Build history of the part. All positions in model axes, mm. Face numbers are marked on the shaded views. A direction names the side the tool comes from. Round coordinates to 2 decimals unless told otherwise and drop trailing zeros. Write each loop counter-clockwise with the first axis right and the second up, starting at its lowest first coordinate (ties: lowest second). Pieces come first, ordered by that corner, then holes.
Item 1: Mould opens along Y. For the marked faces 1, 2 and 3 say: +Y half, -Y half, draft (parallel to the pull), parting line (faces both ways), or undercut.
Item 2: 3-axis set-ups, long thin cutter, end or side, ignore diameter. For the marked faces 4 and 5: which of +Z, -Z, +X, -X, +Y, -Y reach the whole face in a straight line?
Item 3: Band-saw the part on D-D, the plane z = 24.5. Write the cut outline in (x, y) (3 decimals), then the cut area to 3 significant figures.
Item 4: Band-saw the part on A-A, the plane y = -8.5. Write the cut outline in (x, z) (3 decimals).
Item 5: Band-saw the part on B-B, the plane y = 0. Write the cut outline in (x, z) (3 decimals).
Item 6: Band-saw the part on C-C, the plane x = 10. Write the cut outline in (y, z) (3 decimals), then the cut area to 3 significant figures.
Item 7: Drop a flat-ended pin along its axis: pin 1 Ø2 at (x, y) = (-8.5, -17.5) entering from +Z. Give the stop position or say it passes through.
Item 8: Wall check: probe 1 along X at (y, z) = (2, 71.5) (3 decimals); probe 2 along Z at (x, y) = (19.7, 0) (3 decimals). Give the ranges that are in metal, low to high.
```python
from build123d import *

# Parameters (mm, degrees)
SKETCH2_W           = 44.45
SKETCH2_H           = 44.45
SKETCH2_W_2         = 38.1
SKETCH2_H_2         = 38.1
BOSS_EXTRUDE1_DEPTH = 101.6
SKETCH5_R           = 3.175
CUT_EXTRUDE1_DEPTH  = 54.864
CHAMFER1_SIZE       = 12.7


with BuildPart() as part:
    # Sketch2 → Boss-Extrude1 (new body)
    with BuildSketch(Plane.XY):
        Rectangle(SKETCH2_W, SKETCH2_H)
        Rectangle(SKETCH2_W_2, SKETCH2_H_2, mode=Mode.SUBTRACT)
    extrude(amount=BOSS_EXTRUDE1_DEPTH)

    # Sketch5 → Cut-Extrude1 (cut)
    with BuildSketch(Plane.ZY.offset(22.225)):
        with Locations(Location((12.7, 0, 0), (0, 0, 270))):
            Circle(SKETCH5_R)
    extrude(amount=-CUT_EXTRUDE1_DEPTH, mode=Mode.SUBTRACT)

    # Chamfer1
    # the kernel refuses this chamfer: 12.7 mm, written as the material it takes off along each edge
    with BuildSketch(Plane(origin=(54.885373947, -22.225, 0), x_dir=(0, 0.9996219169112966, -0.02749587661058637), z_dir=(-1, 0, 0))) as chamfer1_piece_1:
        Polygon((CHAMFER1_SIZE * 0.999621916911, -CHAMFER1_SIZE * 0.0274958766106), (-CHAMFER1_SIZE * 0.0274958766106, -CHAMFER1_SIZE * 0.999621916911), (0, 0), align=None)
    extrude(amount=109.770747894, mode=Mode.SUBTRACT)
    with BuildSketch(Plane(origin=(-54.885373947, 22.225, 0), x_dir=(0, 0.02749587661058647, 0.9996219169112966), z_dir=(1, 0, 0))) as chamfer1_piece_2:
        Polygon((CHAMFER1_SIZE * 0.999621916911, CHAMFER1_SIZE * 0.0274958766106), (-CHAMFER1_SIZE * 0.0274958766106, CHAMFER1_SIZE * 0.999621916911), (0, 0), align=None)
    extrude(amount=109.770747894, mode=Mode.SUBTRACT)


solid = part.part
```
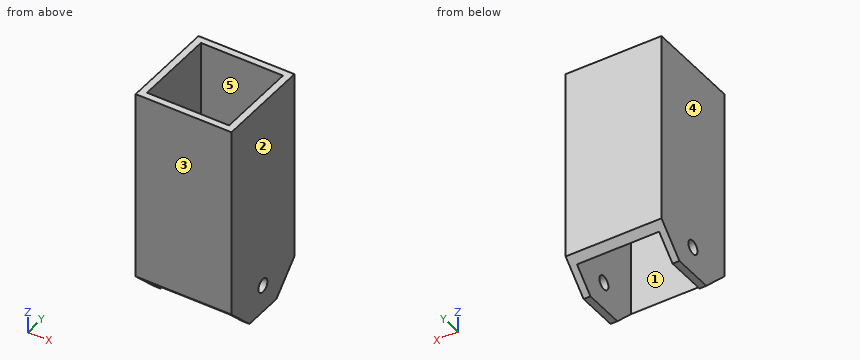
Results:
1. face 1: undercut
1. face 2: draft
1. face 3: -Y half
2. face 4: +Z, -Z, -X, +Y, -Y
2. face 5: +Z, -Z
3. outline: (-22.225, -22.225) - (22.225, -22.225) - (22.225, 22.225) - (-22.225, 22.225) - close; hole (-19.05, -19.05) - (19.05, -19.05) - (19.05, 19.05) - (-19.05, 19.05) - close
3. area: 524 mm2
4. outline: (-22.225, 0) - (-19.05, 0) - (-19.05, 101.6) - (-22.225, 101.6) - close; (19.05, 0) - (22.225, 0) - (22.225, 101.6) - (19.05, 101.6) - close
5. outline: (-22.225, 0) - (-19.05, 0) - (-19.05, 9.525) - (-22.225, 9.525) - close; (-22.225, 15.875) - (-19.05, 15.875) - (-19.05, 101.6) - (-22.225, 101.6) - close; (19.05, 0) - (22.225, 0) - (22.225, 9.525) - (19.05, 9.525) - close; (19.05, 15.875) - (22.225, 15.875) - (22.225, 101.6) - (19.05, 101.6) - close
6. outline: (-22.225, 12.7) - (-19.05, 9.525) - (-19.05, 101.6) - (-22.225, 101.6) - close; (19.05, 9.525) - (22.225, 12.7) - (22.225, 101.6) - (19.05, 101.6) - close
6. area: 575 mm2
7. pin 1: passes through
8. probe 1: x = -22.225 to -19.05, 19.05 to 22.225
8. probe 2: z = 0 to 9.525, 15.875 to 101.6
